from build123d import *

# Parameters (mm, degrees)
SKETCH1_R           = 3.6576
BOSS_EXTRUDE1_DEPTH = 10.287
FILLET1_R           = 0.127
SKETCH2_R           = 1.524
BOSS_EXTRUDE2_DEPTH = 0.762
FILLET2_R           = 0.254
SKETCH3_R           = 0.5461
CUT_EXTRUDE1_DEPTH  = 10.16


with BuildPart() as part:
    # Sketch1 → Boss-Extrude1 (new, symmetric)
    with BuildSketch(Plane(origin=(0, 0, 0), x_dir=(1, 0, 0), z_dir=(0, 1, 0))):
        with Locations(Location((0, 0, 0), (0, 0, 270))):
            Circle(SKETCH1_R)
    extrude(amount=BOSS_EXTRUDE1_DEPTH, both=True)

    # Fillet1
    fillet1_edges = [part.edges().sort_by_distance(p)[0] for p in [
        (0, -10.287, -3.6576),
        (0, 10.287, -3.6576),
    ]]
    fillet(fillet1_edges, radius=FILLET1_R)

    # Sketch2 → Boss-Extrude2 (add)
    with BuildSketch(Plane(origin=(0, 10.287, 0), x_dir=(1, 0, 0), z_dir=(0, 1, 0))):
        with Locations(Location((0, 0, 0), (0, 0, 90))):
            Circle(SKETCH2_R)
    extrude(amount=BOSS_EXTRUDE2_DEPTH)

    # Fillet2
    fillet2_edges = [part.edges().sort_by_distance(p)[0] for p in [
        (0, 11.049, 1.524),
    ]]
    fillet(fillet2_edges, radius=FILLET2_R)

    # Sketch3 → Cut-Extrude1 (cut)
    with BuildSketch(Plane(origin=(0, 11.049, 0), x_dir=(1, 0, 0), z_dir=(0, 1, 0))):
        with Locations(Location((0, 0, 0), (0, 0, 270))):
            Circle(SKETCH3_R)
    extrude(amount=-CUT_EXTRUDE1_DEPTH, mode=Mode.SUBTRACT)


solid = part.part
The listing builds one solid part. Answer for the finished solid, in the listing's coordinates (mm). A direction names the side the tool comes from. Coordinates: 2 decimals unless noted, no trailing zeros. Order: outer loops, then holes, each group sorted by start corner. A loop starts at its lowest first (then second) coordinate and runs counter-clockwise, first axis right, second up. Notation, with made-up numbers: (-35.5, -3) -> (13.5, -3) arc R29 ccw to (13.5, 28) -> close; hole circle Ø10 at (17.25, 30). An arc over 180 degrees is marked (long way). Answer in a Markdown table with one row per item. Add a question column.
Item 1: Which of the six approach directions +Z, -Z, +X, -X, +Y, -Y give full straight-line access (tool end or side, diameter ignored) to faces 1 (the face through (0, -10.287, 0)), 2 (the face through (0, 0.889, 0))?
Item 2: Find section B-B (z = 0). Write down the section's boundary in (x, y) (3 decimals), then the cut area to 3 significant figures.
Item 3: Find section A-A (y = 6). Write down the section's boundary in (x, z).
Item 4: Find section D-D (y = -4.5). Write down the section's boundary in (x, z), then the cut area to 3 significant figures.
Item 5: Find the intervals of material crossed by L1, parallel to X at y = 6, z = 0; L2, parallel to Y at x = -2, z = 1.25; L3, parallel to X at y = -9.25, z = 3.25, in increasing order. Write a range as from..to.
Item 6: Determine the mould class of faces 3 (the face through (0.164, 6.04, 0.521)), 4 (the face through (-1.285, 10.537, -0.819)), 5 (the face through (-2, 10.287, 1)) for opening direction X: +X half, -X half, draft (parallel to the pull), parting line (faces both ways), or undercut.
Item 7: Find section C-C (x = 0). Write down the section's boundary in (y, z) (3 decimals), then the cut area to 3 significant figures.
Result set:
| question | item | result |
|---|---|---|
| 1 | face 1 | +Z, -Z, +X, -X, -Y |
| 1 | face 2 | +Y |
| 2 | outline | (-3.658, -10.16) arc R0.127 ccw to (-3.531, -10.287) -> (3.531, -10.287) arc R0.127 ccw to (3.658, -10.16) -> (3.658, 10.16) arc R0.127 ccw to (3.531, 10.287) -> (1.524, 10.287) -> (1.524, 10.795) arc R0.254 ccw to (1.27, 11.049) -> (0.546, 11.049) -> (0.546, 0.889) -> (-0.546, 0.889) -> (-0.546, 11.049) -> (-1.27, 11.049) arc R0.254 ccw to (-1.524, 10.795) -> (-1.524, 10.287) -> (-3.531, 10.287) arc R0.127 ccw to (-3.658, 10.16) -> close |
| 2 | area | 142 mm² |
| 3 | outline | circle Ø7.32 at (0, 0); hole circle Ø1.09 at (0, 0) |
| 4 | outline | circle Ø7.32 at (0, 0) |
| 4 | area | 42.0 mm² |
| 5 | L1 | x = -3.66..-0.55, 0.55..3.66 |
| 5 | L2 | y = -10.29..10.29 |
| 5 | L3 | x = -1.68..1.68 |
| 6 | face 3 | undercut |
| 6 | face 4 | parting line |
| 6 | face 5 | draft |
| 7 | outline | (-10.287, -3.531) arc R0.127 ccw to (-10.16, -3.658) -> (10.16, -3.658) arc R0.127 ccw to (10.287, -3.531) -> (10.287, -1.524) -> (10.795, -1.524) arc R0.254 ccw to (11.049, -1.27) -> (11.049, -0.546) -> (0.889, -0.546) -> (0.889, 0.546) -> (11.049, 0.546) -> (11.049, 1.27) arc R0.254 ccw to (10.795, 1.524) -> (10.287, 1.524) -> (10.287, 3.531) arc R0.127 ccw to (10.16, 3.658) -> (-10.16, 3.658) arc R0.127 ccw to (-10.287, 3.531) -> close |
| 7 | area | 142 mm² |
